Geometry: final body of the model. Coordinates: model frame, mm. A direction names the side the tool comes from. Round coordinates to 2 decimals unless told otherwise and drop trailing zeros. Order: outer loops, then holes, each group sorted by start corner. A loop starts at its lowest first (then second) coordinate and runs counter-clockwise, first axis right, second up. Notation, with made-up numbers: M 22,2.5 L 70,2.5 A27 cw 70,26.5 Z; hole C -2,-14 d9. An arc over 180 degrees is marked long. Return JSON: item names as keys, results as strings. Group by question number.
Q1. Cut plane D-D on x = 128. Output: boundary loops of the cut face in (y, z), and give its area (3 significant figures).
Q2. Cut plane A-A on x = -80. Output: boundary loops of the cut face in (y, z).
Q3. Contact query for flat-ended pins moving along their axis: pin 1 (1 mm diameter, centred on y = 18, z = 3, fed in from -X); pin 2 (3.5 mm diameter, centred on y = -14.5, z = 3, fed in from +X); pin 3 (1.6 mm diameter, centred on y = -8.5, z = 3.5, fed in from +X); pin 4 (4 mm diameter, centred on x = 15, y = 12.5, fed in from -Z). Output: stop coordinate, or through.
Q4. Cut plane C-C on z = 4.15. Count the separate pieces of the cut face and the enclosed holes in it, and give its area (3 significant figures).
Q5. Access query for faces 4 (the face through (-98.482, 0.813, 2.958)), 5 (the face through (6, 25, 3)). Directions: +Z, -Z, +X, -X, +Y, -Y. A direction counts if a zero-diameter tool reaches every point of the face in a straight line with its end or side. Return the directions, or none.
Q6. Cut plane B-B on x = 8. Output: boundary loops of the cut face in (y, z), and give its area (3 significant figures).
Q7. Ray query, probe 1 along Y at (x, z) = (30.5, 3.1); probe 2 along X at (y, z) = (12, 4.3); probe 3 along X at (y, z) = (10, 1.85). Return the intervals inside material, ascending.
Q8. Mould query, pull axis Y, two halves, no side actions, for faces 1 (the face through (42.5, 12.6, 3)), 2 (the face through (-117.15, 21.99, 2.96)), 3 (the face through (-116.99, -22.15, 2.96)). Classes: released by +Y, released by -Y, zero draft, split by the parting line, or undercut.
```python
from build123d import *

# Parameters (mm, degrees)
ESBO_O1_R                = 18.5
ESBO_O1_R_2              = 4.5
ESBO_O1_R_3              = 4
ESBO_O1_R_4              = 5
ESBO_O1_R_5              = 1.8
ESBO_O1_R_6              = 3
ESBO_O1_R_7              = 1.75
RESSALTO_EXTRUS_O1_DEPTH = 6


with BuildPart() as part:
    # Esboço1 → Ressalto-extrusão1 (new body)
    with BuildSketch(Plane.XY):
        with BuildLine():
            Line((95, -25), (95, -21))
            Line((95, -21), (91.7, -21))
            Line((91.7, -21), (91.7, -17))
            Line((91.7, -17), (95, -17))
            Line((95, -17), (95, -16))
            Line((95, -16), (92.8, -16))
            Line((92.8, -16), (92.8, -13))
            Line((92.8, -13), (91.7, -13))
            Line((91.7, -13), (91.7, -11))
            Line((91.7, -11), (88.3, -11))
            Line((88.3, -11), (88.3, -13))
            Line((88.3, -13), (87.2, -13))
            Line((87.2, -13), (87.2, -16))
            Line((87.2, -16), (85, -16))
            Line((85, -16), (85, -17))
            Line((85, -17), (88.3, -17))
            Line((88.3, -17), (88.3, -21))
            Line((88.3, -21), (85, -21))
            Line((85, -21), (85, -25))
            Line((85, -25), (-32.5, -25))
            Line((-32.5, -25), (-32.5, -21))
            Line((-32.5, -21), (-35.8, -21))
            Line((-35.8, -21), (-35.8, -17))
            Line((-35.8, -17), (-32.5, -17))
            Line((-32.5, -17), (-32.5, -16))
            Line((-32.5, -16), (-34.7, -16))
            Line((-34.7, -16), (-34.7, -13))
            Line((-34.7, -13), (-35.8, -13))
            Line((-35.8, -13), (-35.8, -11))
            Line((-35.8, -11), (-39.2, -11))
            Line((-39.2, -11), (-39.2, -13))
            Line((-39.2, -13), (-40.3, -13))
            Line((-40.3, -13), (-40.3, -16))
            Line((-40.3, -16), (-42.5, -16))
            Line((-42.5, -16), (-42.5, -17))
            Line((-42.5, -17), (-39.2, -17))
            Line((-39.2, -17), (-39.2, -21))
            Line((-39.2, -21), (-42.5, -21))
            Line((-42.5, -21), (-42.5, -25))
            Line((-42.5, -25), (-110, -25))
            ThreePointArc((-110, -25), (-117.071067812, -22.071067812), (-120, -15))
            Line((-120, -15), (-120, 15))
            ThreePointArc((-120, 15), (-117.071067812, 22.071067812), (-110, 25))
            Line((-110, 25), (124.350151348, 25))
            Line((124.350151348, 25), (124.350151348, 27))
            ThreePointArc((124.350151348, 27), (141.627798395, 37.777125853), (143.707891624, 17.520355595))
            Line((143.707891624, 17.520355595), (125, 3))
            Line((125, 3), (125, 0))
            Line((125, 0), (122, 0))
            Line((122, 0), (122, -3.3))
            Line((122, -3.3), (118, -3.3))
            Line((118, -3.3), (118, 0))
            Line((118, 0), (117, 0))
            Line((117, 0), (117, -2.2))
            Line((117, -2.2), (114, -2.2))
            Line((114, -2.2), (114, -3.3))
            Line((114, -3.3), (112, -3.3))
            Line((112, -3.3), (112, -6.7))
            Line((112, -6.7), (114, -6.7))
            Line((114, -6.7), (114, -7.8))
            Line((114, -7.8), (117, -7.8))
            Line((117, -7.8), (117, -10))
            Line((117, -10), (118, -10))
            Line((118, -10), (118, -6.7))
            Line((118, -6.7), (122, -6.7))
            Line((122, -6.7), (122, -10))
            Line((122, -10), (125, -10))
            Line((125, -10), (125, -15))
            ThreePointArc((125, -15), (122.071067812, -22.071067812), (115, -25))
            Line((115, -25), (95, -25))
        make_face()
        with Locations((-80, 0)):
            Circle(ESBO_O1_R, mode=Mode.SUBTRACT)
        with Locations((100, 0)):
            Circle(ESBO_O1_R_2, mode=Mode.SUBTRACT)
        with Locations((136.350151348, 27)):
            Circle(ESBO_O1_R_3, mode=Mode.SUBTRACT)
        with Locations((8, 0)):
            Circle(ESBO_O1_R_4, mode=Mode.SUBTRACT)
        with Locations((-108.81, 0)):
            Circle(ESBO_O1_R_2, mode=Mode.SUBTRACT)
        with Locations((-14.5, 0)):
            Circle(ESBO_O1_R_5, mode=Mode.SUBTRACT)
        with Locations((30.5, 0)):
            Circle(ESBO_O1_R_5, mode=Mode.SUBTRACT)
        with Locations((-29.5, 12.5)):
            Circle(ESBO_O1_R_6, mode=Mode.SUBTRACT)
        with Locations((45.5, 12.5)):
            Circle(ESBO_O1_R_6, mode=Mode.SUBTRACT)
        with Locations((-101.81, 14)):
            Circle(ESBO_O1_R_7, mode=Mode.SUBTRACT)
        with Locations((-101.81, -14)):
            Circle(ESBO_O1_R_7, mode=Mode.SUBTRACT)
    extrude(amount=RESSALTO_EXTRUS_O1_DEPTH)


solid = part.part
```
Result sheet:
{
 "1": {"outline": "M 5.33,0 L 35.62,0 L 35.62,6 L 5.33,6 Z", "area": "182 mm²"},
 "2": {"outline": "M -25,0 L -18.5,0 L -18.5,6 L -25,6 Z; M 18.5,0 L 25,0 L 25,6 L 18.5,6 Z"},
 "3": {"pin 1": "stops at x = -119.68", "pin 2": "stops at x = 125", "pin 3": "stops at x = 122", "pin 4": "stops at z = 0"},
 "4": {"separate pieces": "1", "enclosed holes": "11", "area": "11,100 mm²"},
 "5": {"face 4": "+Z, -Z", "face 5": "+Z, -Z, -X, +Y"},
 "6": {"outline": "M -25,0 L -5,0 L -5,6 L -25,6 Z; M 5,0 L 25,0 L 25,6 L 5,6 Z", "area": "240 mm²"},
 "7": {"probe 1": "y = -25 to -1.8, 1.8 to 25", "probe 2": "x = -120 to -94.08, -65.92 to -32.46, -26.54 to 42.54, 48.46 to 136.6", "probe 3": "x = -120 to -95.56, -64.44 to -31.16, -27.84 to 43.84, 47.16 to 134.02"},
 "8": {"face 1": "undercut", "face 2": "released by +Y", "face 3": "released by -Y"}
}
